```python
from build123d import *

# Parameters (mm, degrees)
BOSS_EXTRUDE2_DEPTH = 8
SKETCH3_R           = 5.25
CUT_EXTRUDE1_DEPTH  = 8
SKETCH7_W           = 4
SKETCH7_H           = 9
BOSS_EXTRUDE3_DEPTH = 8
SKETCH8_W           = 4
SKETCH8_H           = 40
BOSS_EXTRUDE4_DEPTH = 12
SKETCH9_W           = 20
SKETCH9_H           = 4
BOSS_EXTRUDE5_DEPTH = 24
SKETCH10_W          = 20
SKETCH10_H          = 4
BOSS_EXTRUDE6_DEPTH = 24
SKETCH12_W          = 4
SKETCH12_H          = 38
BOSS_EXTRUDE7_DEPTH = 20
SKETCH13_W          = 4
SKETCH13_H          = 20
BOSS_EXTRUDE8_DEPTH = 12
SKETCH14_R          = 1.5
CUT_EXTRUDE2_DEPTH  = 12
SKETCH15_R          = 1.5
CUT_EXTRUDE3_DEPTH  = 12
FILLET1_R           = 3
SKETCH16_R          = 1.5
CUT_EXTRUDE4_DEPTH  = 12


with BuildPart() as part:
    # Sketch1 → Boss-Extrude2 (new body)
    with BuildSketch(Plane.XY):
        with BuildLine():
            ThreePointArc((12, 11), (1, 0), (12, -11))
            Line((12, -11), (12, 11))
        make_face()
        with BuildLine():
            Line((12, 11), (12, -11))
            ThreePointArc((12, -11), (19.778174593, -7.778174593), (23, 0))
            ThreePointArc((23, 0), (19.778174593, 7.778174593), (12, 11))
        make_face()
        with BuildLine():
            Line((-12, 11), (-12, -11))
            Line((-12, -11), (12, -11))
            ThreePointArc((12, -11), (1, 0), (12, 11))
            Line((12, 11), (-12, 11))
        make_face()
    extrude(amount=BOSS_EXTRUDE2_DEPTH)

    # Sketch3 → Cut-Extrude1 (cut)
    with BuildSketch(Plane.XY.offset(8)):
        with Locations((12, 0)):
            Circle(SKETCH3_R)
    extrude(amount=-CUT_EXTRUDE1_DEPTH, mode=Mode.SUBTRACT)

    # Sketch7 → Boss-Extrude3 (add)
    with BuildSketch(Plane.XY.offset(8)):
        with Locations((-10, 15.5)):
            Rectangle(SKETCH7_W, SKETCH7_H)
        with Locations((-10, -15.5)):
            Rectangle(SKETCH7_W, SKETCH7_H)
    extrude(amount=-BOSS_EXTRUDE3_DEPTH)

    # Sketch8 → Boss-Extrude4 (add)
    with BuildSketch(Plane(origin=(0, 0, 0), x_dir=(-1, 0, 0), z_dir=(0, 0, -1))):
        with Locations((10, 0)):
            Rectangle(SKETCH8_W, SKETCH8_H)
    extrude(amount=BOSS_EXTRUDE4_DEPTH)

    # Sketch9 → Boss-Extrude5 (add)
    with BuildSketch(Plane.ZY.offset(12)):
        with Locations((-2, 18)):
            Rectangle(SKETCH9_W, SKETCH9_H)
    extrude(amount=BOSS_EXTRUDE5_DEPTH)

    # Sketch10 → Boss-Extrude6 (add)
    with BuildSketch(Plane.ZY.offset(12)):
        with Locations((-2, -18)):
            Rectangle(SKETCH10_W, SKETCH10_H)
    extrude(amount=BOSS_EXTRUDE6_DEPTH)

    # Sketch12 → Boss-Extrude7 (add)
    with BuildSketch(Plane(origin=(0, 0, -12), x_dir=(-1, 0, 0), z_dir=(0, 0, -1))):
        with Locations((34, 39)):
            Rectangle(SKETCH12_W, SKETCH12_H)
    extrude(amount=-BOSS_EXTRUDE7_DEPTH)

    # Sketch13 → Boss-Extrude8 (add)
    with BuildSketch(Plane.XZ.offset(20)):
        with Locations((-34, -2)):
            Rectangle(SKETCH13_W, SKETCH13_H)
    extrude(amount=BOSS_EXTRUDE8_DEPTH)

    # Sketch14 → Cut-Extrude2 (cut)
    with BuildSketch(Plane.ZY.offset(36)):
        with Locations((-2, -27.5)):
            Circle(SKETCH14_R)
    extrude(amount=-CUT_EXTRUDE2_DEPTH, mode=Mode.SUBTRACT)

    # Sketch15 → Cut-Extrude3 (cut)
    with BuildSketch(Plane.ZY.offset(36)):
        with Locations((-2, 51)):
            Circle(SKETCH15_R)
        with Locations((-2, 44)):
            Circle(SKETCH15_R)
        with Locations((-2, 37)):
            Circle(SKETCH15_R)
        with Locations((-2, 30)):
            Circle(SKETCH15_R)
    extrude(amount=-CUT_EXTRUDE3_DEPTH, mode=Mode.SUBTRACT)

    # Fillet1
    fillet1_edges = [part.edges().sort_by_distance(p)[0] for p in [
        (-34, -32, -12),
        (-34, -32, 8),
        (-34, 58, 8),
        (-34, 58, -12),
    ]]
    fillet(fillet1_edges, radius=FILLET1_R)

    # Sketch16 → Cut-Extrude4 (cut)
    with BuildSketch(Plane(origin=(0, 0, 0), x_dir=(-1, 0, 0), z_dir=(0, 0, -1))):
        with Locations((-12, 8.5)):
            Circle(SKETCH16_R)
        with Locations((-20.5, 0)):
            Circle(SKETCH16_R)
        with Locations((-12, -8.5)):
            Circle(SKETCH16_R)
        with Locations((-3.5, 0)):
            Circle(SKETCH16_R)
    extrude(amount=-CUT_EXTRUDE4_DEPTH, mode=Mode.SUBTRACT)


solid = part.part
```
CAD build for the part. Positions are in the model's coordinates, mm. A direction names the side the tool comes from. Round coordinates to 2 decimals unless told otherwise and drop trailing zeros. Order: outer loops, then holes, each group sorted by start corner. A loop starts at its lowest first (then second) coordinate and runs counter-clockwise, first axis right, second up.
Item 1: Saw through at C-C on z = -1.5. State how many separate pieces and enclosed holes the cut face has, then the cut area to 3 significant figures.
Item 2: Probe line 1 along Y through (x, z) = (-26.5, -5.75); line 2 along X through (y, z) = (19.5, 3.25); line 3 along Z through (x, y) = (3, -10). List the from-to ranges inside material, lowest first.
Item 3: Tool access for faces 1 (the face through (2, -11, 4)), 2 (the face through (4, 3, 0)), 3 (the face through (2, 11, 4)), 4 (the face through (-12, 0, -2)): list every direction of +Z, -Z, +X, -X, +Y, -Y with a clear straight run to the whole face (end or side of a thin tool).
Item 4: Saw through at B-B on y = -27.5. Write the cut outline in (x, z).
Item 5: Saw through at A-A on x = -22.5. Write the cut outline in (y, z), then the cut area to 3 significant figures.
Item 6: Mould opens along X. For faces 5 (the face through (-24, -16, -2)), 6 (the face through (13.2, 7.6, 3.9)), 7 (the face through (-8, 0, -4)), 8 (the face through (13.2, -9.4, 3.9)) say: pulls with the +X half, pulls with the -X half, needs draft (parallel to the pull), parting line crosses it, or undercut.
Item 7: Saw through at D-D on z = -7. Write the cut outline in (x, y).
Item 8: Pin check, flat tips, straight feed: pin 1 (8 mm diameter, centred on x = -17.5, y = 27.5, fed in from -Z); pin 2 (10 mm diameter, centred on x = -25, z = 3, fed in from -Y); pin 3 (4 mm diameter, centred on x = 6.5, z = 5, fed in from -Y); pin 4 (4 mm diameter, centred on x = 0.5, z = 4, fed in from +Y). Stop position of each tip, or through.
Reported:
1. separate pieces: 6
1. enclosed holes: 0
1. area: 495 mm2
2. line 1: y = -20 to -16, 16 to 20
2. line 2: x = -36 to -8
2. line 3: z = 0 to 8
3. face 1: +Z, -Z, +X, -Y
3. face 2: -Z, +X, +Y, -Y
3. face 3: +Z, -Z, +X, +Y
3. face 4: +Z, -Z, -X
4. outline: (-36, -12) - (-32, -12) - (-32, -3.5) - (-36, -3.5) - close; (-36, -0.5) - (-32, -0.5) - (-32, 8) - (-36, 8) - close
5. outline: (-20, -12) - (-16, -12) - (-16, 8) - (-20, 8) - close; (16, -12) - (20, -12) - (20, 8) - (16, 8) - close
5. area: 160 mm2
6. face 5: needs draft
6. face 6: undercut
6. face 7: pulls with the +X half
6. face 8: undercut
7. outline: (-36, -32) - (-32, -32) - (-32, -20) - (-8, -20) - (-8, 20) - (-32, 20) - (-32, 58) - (-36, 58) - (-36, 16) - (-12, 16) - (-12, -16) - (-36, -16) - close
8. pin 1: passes through
8. pin 2: stops at y = -20
8. pin 3: stops at y = -11
8. pin 4: stops at y = 11
